```python
from build123d import *

# Parameters (mm, degrees)
BOSS_EXTRUDE1_DEPTH    = 25
CUT_EXTRUDE1_REACH     = 37.102
SKETCH2_R              = 2.25
CUT_EXTRUDE2_REACH     = 37.892
SKETCH3_R              = 2.25
CONVERT_SOLID1_START   = -25
CONVERT_SOLID1_DEPTH   = 50
CONVERT_SOLID1_2_DEPTH = 50


# Read off the part's stored shape, not the designer's step: Convert-Solid1
with BuildPart() as part:
    # Sketch1 → Boss-Extrude1 (new, symmetric)
    with BuildSketch(Plane(origin=(0, 0, 0), x_dir=(0, 0, -1), z_dir=(1, 0, 0))):
        Polygon((0, 0), (-16.884776311, 16.884776311), (-15.824116139, 17.945436483), (3.621320344, -1.5), (-16.378679656, -1.5), (-16.378679656, 0), align=None)
    extrude(amount=BOSS_EXTRUDE1_DEPTH, both=True)

    # Sketch2 → Cut-Extrude1 (cut, up to next)
    with BuildSketch(Plane(origin=(0, 1.060660172, -1.060660172), x_dir=(1, 0, 0), z_dir=(0, 0.7071067811865513, -0.7071067811865438)), mode=Mode.PRIVATE) as cut_extrude1_sk1:
        with Locations(Location((-15, -16.378679656, 0), (0, 0, 270))):
            Circle(SKETCH2_R)
    cut_extrude1_tool1 = extrude(cut_extrude1_sk1.sketch, amount=-CUT_EXTRUDE1_REACH, mode=Mode.PRIVATE) & part.part
    # Sketch2 → Cut-Extrude1 (cut, up to next)
    with BuildSketch(Plane(origin=(0, 1.060660172, -1.060660172), x_dir=(1, 0, 0), z_dir=(0, 0.7071067811865513, -0.7071067811865438)), mode=Mode.PRIVATE) as cut_extrude1_sk2:
        with Locations(Location((15, -16.378679656, 0), (0, 0, 270))):
            Circle(SKETCH2_R)
    cut_extrude1_tool2 = extrude(cut_extrude1_sk2.sketch, amount=-CUT_EXTRUDE1_REACH, mode=Mode.PRIVATE) & part.part
    add(cut_extrude1_tool1.solids().sort_by_distance((-15, 12.642136, 10.520815))[0], mode=Mode.SUBTRACT)
    add(cut_extrude1_tool2.solids().sort_by_distance((15, 12.642136, 10.520815))[0], mode=Mode.SUBTRACT)

    # Sketch3 → Cut-Extrude2 (cut, up to next)
    with BuildSketch(Plane.XZ.offset(1.5), mode=Mode.PRIVATE) as cut_extrude2_sk1:
        with Locations(Location((-15, 8.878679656, 0), (0, 0, 270))):
            Circle(SKETCH3_R)
    cut_extrude2_tool1 = extrude(cut_extrude2_sk1.sketch, amount=-CUT_EXTRUDE2_REACH, mode=Mode.PRIVATE) & part.part
    # Sketch3 → Cut-Extrude2 (cut, up to next)
    with BuildSketch(Plane.XZ.offset(1.5), mode=Mode.PRIVATE) as cut_extrude2_sk2:
        with Locations(Location((15, 8.878679656, 0), (0, 0, 270))):
            Circle(SKETCH3_R)
    cut_extrude2_tool2 = extrude(cut_extrude2_sk2.sketch, amount=-CUT_EXTRUDE2_REACH, mode=Mode.PRIVATE) & part.part
    add(cut_extrude2_tool1.solids().sort_by_distance((-15, -1.5, 8.87868))[0], mode=Mode.SUBTRACT)
    add(cut_extrude2_tool2.solids().sort_by_distance((15, -1.5, 8.87868))[0], mode=Mode.SUBTRACT)

    # Convert-Solid1 outline → Convert-Solid1 (cut)
    with BuildSketch(Plane.YZ.offset(CONVERT_SOLID1_START)):
        with BuildLine():
            Line((-1.5, -3.621320344), (4.474873734, 2.353553391))
            ThreePointArc((4.474873734, 2.353553391), (3.048097173, 1.489042104), (1.383203961, 1.383203961))
            Line((1.383203961, 1.383203961), (0, 0))
            Line((0, 0), (0, 1.956145802))
            ThreePointArc((0, 1.956145802), (-1.102418412, 3.20824195), (-1.5, 4.828427125))
            Line((-1.5, 4.828427125), (-1.5, -3.621320344))
        make_face()
    extrude(amount=CONVERT_SOLID1_DEPTH, mode=Mode.SUBTRACT)

    # Convert-Solid1 2 outline → Convert-Solid1 2 (add)
    with BuildSketch(Plane.YZ.offset(CONVERT_SOLID1_START)):
        with BuildLine():
            ThreePointArc((0, 1.956145802), (0.660607987, 1.594848761), (1.383203961, 1.383203961))
            Line((1.383203961, 1.383203961), (3.414213562, 3.414213562))
            ThreePointArc((3.414213562, 3.414213562), (1.234633135, 2.98066806), (0, 4.828427125))
            Line((0, 4.828427125), (0, 1.956145802))
        make_face()
    extrude(amount=CONVERT_SOLID1_2_DEPTH)


solid = part.part
```
Check sheet for the modelled part. Datum: model origin and axes. Units: mm. A direction names the side the tool comes from. Give positions to 0.01 mm unless a question says otherwise; leave off trailing zeros. Write each loop counter-clockwise with the first axis right and the second up, starting at its lowest first coordinate (ties: lowest second). Pieces come first, ordered by that corner, then holes. Notation, with made-up numbers: (89.5, 55.25) -> (148.5, 55.25) arc R17 cw to (148.5, 74.25) -> close; hole circle Ø10 at (35.5, 28.5). An arc over 180 degrees is marked (long way). Use CSV: the item, a comma, the result in double quotes. Start each with the question number.
Q1. Cross-section at D-D on y = -0.5. Enter the section's corners in (x, z), and give its area (3 significant figures).
Q2. Release check for a two-part mould opening along X. For faces 1 (the flat face through (0.35, 17.41, 16.36)), 2 (the flat face through (25, 7.5, 6.8)), 3 (the cylindrical face through (12.8, 11.8, 10.7)) record: +X half, -X half, draft (parallel to the pull), parting line (faces both ways), or undercut.
Q3. Cross-section at C-C on x = -15. Enter the section's corners in (y, z).
Q4. Cross-section at B-B on z = 4. Enter the section's corners in (x, y), and give its area (3 significant figures).
Q5. Scan lines: line 1 along Y through (x, z) = (16, 14.25); line 2 along Y through (x, z) = (19.5, 16); line 3 along Z through (x, y) = (-17.5, 14.5). Record each from-to range of solid material in increasing order.
Q6. Tool access check on faces 4 (the flat face through (0, -1, 16.379)), 5 (the cylindrical face through (12.804, -0.76, 9.366)), 6 (the flat face through (0, 10, 10)). Record the directions out of +Z, -Z, +X, -X, +Y, -Y that give a thin tool (end or side, any length) a straight path to the whole face; none if there is none.
Q7. Cross-section at A-A on x = 7. Enter the section's corners in (y, z), and give its area (3 significant figures).
Q8. Depth check by flat-ended pin: P1, Ø5, axis at x = 15, z = 8.88, coming from the +Y side; P2, Ø10, axis at x = -15.5, y = 11, coming from the +Z side; P3, Ø6, axis at x = 12, z = 8.5, coming from the +Y side. Enter the tip coordinate at first touch or a pass-through.
Working result:
1,outline,"(-25, 2.38) -> (25, 2.38) -> (25, 16.38) -> (-25, 16.38) -> close; hole circle Ø4.5 at (-15, 8.88); hole circle Ø4.5 at (15, 8.88)"
1,area,"668 mm^2"
2,face 1,"draft"
2,face 2,"+X half"
2,face 3,"undercut"
3,outline,"(-1.5, 4.83) arc R3.5 ccw to (4.47, 2.35) -> (11.05, 8.93) -> (9.99, 9.99) -> (3.41, 3.41) arc R2 cw to (0, 4.83) -> (0, 6.63) -> (-1.5, 6.63) -> close; (-1.5, 11.13) -> (0, 11.13) -> (0, 16.38) -> (-1.5, 16.38) -> close; (13.17, 13.17) -> (14.23, 12.11) -> (17.95, 15.82) -> (16.88, 16.88) -> close"
4,outline,"(-25, -1.4) -> (25, -1.4) -> (25, 0.18) -> (-25, 0.18) -> close; (-25, 4) -> (25, 4) -> (25, 6.12) -> (-25, 6.12) -> close"
4,area,"185 mm^2"
5,line 1,"y = -1.5 to 0, 14.25 to 16.37"
5,line 2,"y = -1.5 to 0, 16 to 17.77"
5,line 3,"z = 12.38 to 14.5"
6,face 4,"+Z, +X, -X, -Y"
6,face 5,"-Y"
6,face 6,"+Z, +X, -X"
7,outline,"(-1.5, 4.83) arc R3.5 ccw to (4.47, 2.35) -> (17.95, 15.82) -> (16.88, 16.88) -> (3.41, 3.41) arc R2 cw to (0, 4.83) -> (0, 16.38) -> (-1.5, 16.38) -> close"
7,area,"55.6 mm^2"
8,P1,"stops at y = 12.23"
8,P2,"stops at z = 16"
8,P3,"stops at y = 13.62"
